```python
from build123d import *

# Parameters (mm, degrees)
SKETCH_1_R               = 13
EXTRUDE_1_DEPTH          = 2
SKETCH_2_R               = 13
SKETCH_2_R_2             = 10
EXTRUDE_2_DEPTH          = 5
SKETCH_4_R               = 25
SKETCH_4_R_2             = 10
EXTRUDE_3_DEPTH          = 1
SKETCH_5_R               = 22.5
SKETCH_5_R_2             = 10
EXTRUDE_4_DEPTH          = 10
SKETCH_6_R               = 1.25
CUT_EXTRUDE_1_DEPTH      = 8
SKETCH_7_R               = 3
SKETCH_7_R_2             = 1
CUT_EXTRUDE_2_DEPTH      = 40.67366885
CUT_EXTRUDE_3_DEPTH      = 40.67366885
CUT_EXTRUDE_3_DEPTH_BACK = 40.67366885
SKETCH_8_W               = 14
SKETCH_8_H               = 5


with BuildPart() as part:
    # 스케치1 → 보스-돌출1 (new body)
    with BuildSketch(Plane.XY):
        Circle(SKETCH_1_R)
    extrude(amount=EXTRUDE_1_DEPTH)

    # 스케치2 → 보스-돌출2 (add)
    with BuildSketch(Plane.XY.offset(2)):
        Circle(SKETCH_2_R)
        Circle(SKETCH_2_R_2, mode=Mode.SUBTRACT)
    extrude(amount=EXTRUDE_2_DEPTH)

    # 스케치4 → 보스-돌출3 (add)
    with BuildSketch(Plane.XY.offset(7)):
        Circle(SKETCH_4_R)
        Circle(SKETCH_4_R_2, mode=Mode.SUBTRACT)
    extrude(amount=EXTRUDE_3_DEPTH)

    # 스케치5 → 보스-돌출4 (add)
    with BuildSketch(Plane.XY.offset(8)):
        Circle(SKETCH_5_R)
        Circle(SKETCH_5_R_2, mode=Mode.SUBTRACT)
    extrude(amount=EXTRUDE_4_DEPTH)

    # 스케치6 → 컷-돌출1 (cut)
    with BuildSketch(Plane.XY.offset(18)):
        with Locations((0, 18.75)):
            Circle(SKETCH_6_R)
        with Locations((18.75, 0)):
            Circle(SKETCH_6_R)
        with Locations((13.258252147, -13.258252147)):
            Circle(SKETCH_6_R)
        with Locations((0, -18.75)):
            Circle(SKETCH_6_R)
        with Locations((-13.258252147, -13.258252147)):
            Circle(SKETCH_6_R)
        with Locations((-18.75, 0)):
            Circle(SKETCH_6_R)
    extrude(amount=-CUT_EXTRUDE_1_DEPTH, mode=Mode.SUBTRACT)

    # 스케치7 → 컷-돌출2 (cut, through all)
    with BuildSketch(Plane(origin=(0, 0, 0), x_dir=(-1, 0, 0), z_dir=(0, 0, -1))):
        Circle(SKETCH_7_R)
        with Locations((0, 7)):
            Circle(SKETCH_7_R_2)
        with Locations((0, -7)):
            Circle(SKETCH_7_R_2)
        with Locations((-7, 3)):
            Circle(SKETCH_7_R_2)
        with Locations((-7, -3)):
            Circle(SKETCH_7_R_2)
        with Locations((7, 3)):
            Circle(SKETCH_7_R_2)
        with Locations((7, -3)):
            Circle(SKETCH_7_R_2)
    extrude(amount=-CUT_EXTRUDE_2_DEPTH, mode=Mode.SUBTRACT)

    # 스케치8 → 컷-돌출3 (cut, two sides: drawn at the far end of the back side and taken through both)
    with BuildSketch(Plane(origin=(0, 0, 0), x_dir=(1, 0, 0), z_dir=(0, 1, 0)).offset(-CUT_EXTRUDE_3_DEPTH_BACK)):
        with Locations((0, -4.5)):
            Rectangle(SKETCH_8_W, SKETCH_8_H)
    extrude(amount=CUT_EXTRUDE_3_DEPTH + CUT_EXTRUDE_3_DEPTH_BACK, mode=Mode.SUBTRACT)


solid = part.part
```
Read the model definition and answer for the solid it produces. Units are mm, in the model's axes. A direction names the side the tool comes from. Coordinates: 2 decimals unless noted, no trailing zeros. Write each loop counter-clockwise with the first axis right and the second up, starting at its lowest first coordinate (ties: lowest second). Pieces come first, ordered by that corner, then holes. Notation, with made-up numbers: (-2.75, 84) - (47.25, 84) arc R23 ccw to (47.25, 119) - close; hole circle Ø11 at (89.25, 16.5). An arc over 180 degrees is marked (long way). Answer as a JSON object with one key per item and string values. Group by question number.
1. Which of the six approach directions +Z, -Z, +X, -X, +Y, -Y give full straight-line access (tool end or side, diameter ignored) to faces 3 (the cylindrical face through (12.01, -13.2, 14.06)), 4 (the flat face through (-7, 9, 5)), 5 (the flat face through (-0.3, 10.3, 18))?
2. A cutting plane is placed at C-C (x = 5). Determine the outline of the cut face in (y, z), plus the area to 3 significant figures.
3. A cutting plane is placed at D-D (z = 9). Determine the outline of the cut face in (x, y), plus the area to 3 significant figures.
4. Each of these flat-tipped pins is pushed along its axis until it touches: P1, Ø2, axis at x = 6, y = -6.5, coming from the -Z side; P2, Ø4, axis at y = 8.5, z = 4, coming from the -X side; P3, Ø2, axis at x = 0, y = 18.75, coming from the +Z side; P4, Ø1, axis at x = 14, z = 14, coming from the +Y side. Where does it stop, or does it pass through?
5. A cutting plane is placed at A-A (y = 0). Determine the outline of the cut face in (x, z).
6. Consider L1, parallel to Y at x = 0, z = 1.25; L2, parallel to Y at x = 0, z = 14; L3, parallel to Y at x = -7, z = 1.25. Determine where each line is inside the solid, lowest interval first. Write a range as [from, to].
7. A cutting plane is placed at B-B (z = 6). Determine the outline of the cut face in (x, y).
8. The mould has two halves that part along X. Classify faces 1 (the flat face through (3, -3, 0)), 2 (the flat face through (-7, -9, 5)): +X half, -X half, draft (parallel to the pull), parting line (faces both ways), or undercut.
Worked out:
{
 "1": {"face 3": "+Z", "face 4": "+Y, -Y", "face 5": "+Z, +X, -X, +Y, -Y"},
 "2": {"outline": "(-24.49, 7) - (-8.66, 7) - (-8.66, 18) - (-21.94, 18) - (-21.94, 8) - (-24.49, 8) - close; (-12, 0) - (12, 0) - (12, 2) - (-12, 2) - close; (8.66, 7) - (24.49, 7) - (24.49, 8) - (21.94, 8) - (21.94, 18) - (8.66, 18) - close", "area": "345 mm²"},
 "3": {"outline": "circle Ø45 at (0, 0); hole circle Ø20 at (0, 0)", "area": "1,280 mm²"},
 "4": {"P1": "stops at z = 0", "P2": "stops at x = -11.26", "P3": "stops at z = 10", "P4": "stops at y = 18"},
 "5": {"outline": "(-25, 7) - (-13, 7) - (-13, 0) - (-3, 0) - (-3, 2) - (-10, 2) - (-10, 18) - (-17.5, 18) - (-17.5, 10) - (-20, 10) - (-20, 18) - (-22.5, 18) - (-22.5, 8) - (-25, 8) - close; (3, 0) - (13, 0) - (13, 7) - (25, 7) - (25, 8) - (22.5, 8) - (22.5, 18) - (20, 18) - (20, 10) - (17.5, 10) - (17.5, 18) - (10, 18) - (10, 2) - (3, 2) - close"},
 "6": {"L1": "y = [-13, -8], [-6, -3], [3, 6], [8, 13]", "L2": "y = [-22.5, -20], [-17.5, -10], [10, 17.5], [20, 22.5]", "L3": "y = [-10.95, -4], [-2, 2], [4, 10.95]"},
 "7": {"outline": "(-7, -10.95) - (-7, -7.14) arc R10 cw to (-7, 7.14) - (-7, 10.95) arc R13 ccw to start; (7, -10.95) arc R13 ccw to (7, 10.95) - (7, 7.14) arc R10 cw to (7, -7.14) - close"},
 "8": {"face 1": "draft", "face 2": "undercut"}
}
